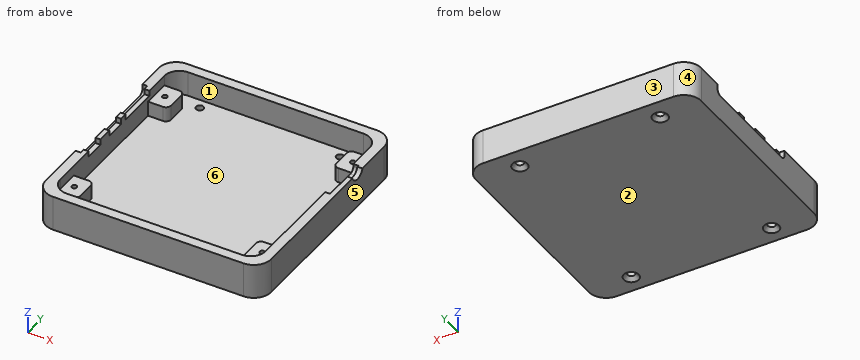
from build123d import *

# Parameters (mm, degrees)
CYLINDER005_R     = 1
CYLINDER005_DEPTH = 8
BOX014_W          = 8
BOX014_H          = 11
BOX014_DEPTH      = 6
FILLET006_R       = 2
CYLINDER006_R     = 1
CYLINDER006_DEPTH = 9
BOX013_W          = 8
BOX013_H          = 11
BOX013_DEPTH      = 6
FILLET005_R       = 2
CYLINDER004_R     = 1
CYLINDER004_DEPTH = 8
BOX011_W          = 8
BOX011_H          = 11
BOX011_DEPTH      = 6
FILLET004_R       = 2
CYLINDER003_R     = 1
CYLINDER003_DEPTH = 8
BOX009_W          = 8
BOX009_H          = 11
BOX009_DEPTH      = 6
FILLET003_R       = 2
BOX024_W          = 2
BOX024_H          = 45
BOX024_DEPTH      = 8
FILLET007_R       = 2
BOX023_W          = 6
BOX023_H          = 8
BOX023_DEPTH      = 3
CYLINDER008_R     = 1.5
CYLINDER008_DEPTH = 10
CYLINDER009_R     = 1.5
CYLINDER009_DEPTH = 10
CYLINDER010_R     = 1.5
CYLINDER010_DEPTH = 10
CYLINDER007_R     = 1.5
CYLINDER007_DEPTH = 10
BOX018_W          = 6
BOX018_H          = 8
BOX018_DEPTH      = 3
BOX015_W          = 16
BOX015_H          = 16
BOX015_DEPTH      = 2.25
CYLINDER002_R     = 3.5
CYLINDER002_DEPTH = 10.5
BOX010_W          = 2
BOX010_H          = 19
BOX010_DEPTH      = 8
FILLET002_R       = 2
BOX008_W          = 90
BOX008_H          = 90
BOX008_DEPTH      = 14
BOX006_W          = 82
BOX006_H          = 82
BOX006_DEPTH      = 82
FILLET001_R       = 6
BOX005_W          = 90
BOX005_H          = 90
BOX005_DEPTH      = 90
FILLET_R          = 7
CHAMFER_SIZE      = 1.5


with BuildPart() as cylinder002:
    # Cylinder005 → Cylinder005 (new body)
    with BuildSketch(Plane(origin=(82.5, 74.5, 4), x_dir=(1, 0, 0), z_dir=(0, 0, 1))):
        Circle(CYLINDER005_R)
    extrude(amount=CYLINDER005_DEPTH)


with BuildPart() as cut003:
    # Box014 → Box014 (new body)
    with BuildSketch(Plane(origin=(78, 8, 4), x_dir=(1, 0, 0), z_dir=(0, 0, 1))):
        with Locations((4, 5.5)):
            Rectangle(BOX014_W, BOX014_H)
    extrude(amount=BOX014_DEPTH)

    # Fillet006
    fillet006_edges = [cut003.edges().sort_by_distance(p)[0] for p in [
        (78, 8, 7),
        (78, 19, 7),
    ]]
    fillet(fillet006_edges, radius=FILLET006_R)


with BuildPart() as cut003_1:
    # Fillet006 placement: moved
    add(cut003.part.moved(Location((0, 61, 0))))

    # Cut003: cut Cylinder002
    add(cylinder002.part, mode=Mode.SUBTRACT)


with BuildPart() as cylinder003:
    # Cylinder006 → Cylinder006 (new body)
    with BuildSketch(Plane(origin=(82.5, 13.5, 4), x_dir=(1, 0, 0), z_dir=(0, 0, 1))):
        Circle(CYLINDER006_R)
    extrude(amount=CYLINDER006_DEPTH)


with BuildPart() as cut004:
    # Box013 → Box013 (new body)
    with BuildSketch(Plane(origin=(78, 8, 4), x_dir=(1, 0, 0), z_dir=(0, 0, 1))):
        with Locations((4, 5.5)):
            Rectangle(BOX013_W, BOX013_H)
    extrude(amount=BOX013_DEPTH)

    # Fillet005
    fillet005_edges = [cut004.edges().sort_by_distance(p)[0] for p in [
        (78, 8, 7),
        (78, 19, 7),
    ]]
    fillet(fillet005_edges, radius=FILLET005_R)

    # Cut004: cut Cylinder003
    add(cylinder003.part, mode=Mode.SUBTRACT)


with BuildPart() as cylinder001:
    # Cylinder004 → Cylinder004 (new body)
    with BuildSketch(Plane(origin=(7.5, 74.5, 4), x_dir=(1, 0, 0), z_dir=(0, 0, 1))):
        Circle(CYLINDER004_R)
    extrude(amount=CYLINDER004_DEPTH)


with BuildPart() as cut005:
    # Box011 → Box011 (new body)
    with BuildSketch(Plane(origin=(4, 8, 3), x_dir=(1, 0, 0), z_dir=(0, 0, 1))):
        with Locations((4, 5.5)):
            Rectangle(BOX011_W, BOX011_H)
    extrude(amount=BOX011_DEPTH)

    # Fillet004
    fillet004_edges = [cut005.edges().sort_by_distance(p)[0] for p in [
        (12, 8, 6),
        (12, 19, 6),
    ]]
    fillet(fillet004_edges, radius=FILLET004_R)


with BuildPart() as cut005_1:
    # Fillet004 placement: moved
    add(cut005.part.moved(Location((0, 61, 1))))

    # Cut005: cut Cylinder001
    add(cylinder001.part, mode=Mode.SUBTRACT)


with BuildPart() as cylinder:
    # Cylinder003 → Cylinder003 (new body)
    with BuildSketch(Plane(origin=(7.5, 13.5, 4), x_dir=(1, 0, 0), z_dir=(0, 0, 1))):
        Circle(CYLINDER003_R)
    extrude(amount=CYLINDER003_DEPTH)


with BuildPart() as cut006:
    # Box009 → Box009 (new body)
    with BuildSketch(Plane(origin=(4, 8, 3), x_dir=(1, 0, 0), z_dir=(0, 0, 1))):
        with Locations((4, 5.5)):
            Rectangle(BOX009_W, BOX009_H)
    extrude(amount=BOX009_DEPTH)

    # Fillet003
    fillet003_edges = [cut006.edges().sort_by_distance(p)[0] for p in [
        (12, 8, 6),
        (12, 19, 6),
    ]]
    fillet(fillet003_edges, radius=FILLET003_R)


with BuildPart() as cut006_1:
    # Fillet003 placement: moved
    add(cut006.part.moved(Location((0, 0, 1))))

    # Cut006: cut Cylinder
    add(cylinder.part, mode=Mode.SUBTRACT)


with BuildPart() as fillet007:
    # Box024 → Box024 (new body)
    with BuildSketch(Plane(origin=(0, 27, 10), x_dir=(1, 0, 0), z_dir=(0, 0, 1))):
        with Locations((1, 22.5)):
            Rectangle(BOX024_W, BOX024_H)
    extrude(amount=BOX024_DEPTH)

    # Fillet007
    fillet007_edges = [fillet007.edges().sort_by_distance(p)[0] for p in [
        (1, 27, 10),
        (1, 27, 18),
        (1, 72, 10),
        (1, 72, 18),
    ]]
    fillet(fillet007_edges, radius=FILLET007_R)


with BuildPart() as uart001:
    # Box023 → Box023 (new body)
    with BuildSketch(Plane(origin=(0, 43, 11.75), x_dir=(1, 0, 0), z_dir=(0, 0, 1))):
        with Locations((3, 4)):
            Rectangle(BOX023_W, BOX023_H)
    extrude(amount=BOX023_DEPTH)


with BuildPart() as cylinder005:
    # Cylinder008 → Cylinder008 (new body)
    with BuildSketch(Plane(origin=(17, 7, 0), x_dir=(1, 0, 0), z_dir=(0, 0, 1))):
        Circle(CYLINDER008_R)
    extrude(amount=CYLINDER008_DEPTH)


with BuildPart() as cylinder006:
    # Cylinder009 → Cylinder009 (new body)
    with BuildSketch(Plane(origin=(17, 82, 0), x_dir=(1, 0, 0), z_dir=(0, 0, 1))):
        Circle(CYLINDER009_R)
    extrude(amount=CYLINDER009_DEPTH)


with BuildPart() as cylinder007:
    # Cylinder010 → Cylinder010 (new body)
    with BuildSketch(Plane(origin=(73, 82, 0), x_dir=(1, 0, 0), z_dir=(0, 0, 1))):
        Circle(CYLINDER010_R)
    extrude(amount=CYLINDER010_DEPTH)


with BuildPart() as cylinder004:
    # Cylinder007 → Cylinder007 (new body)
    with BuildSketch(Plane(origin=(73, 7, 0), x_dir=(1, 0, 0), z_dir=(0, 0, 1))):
        Circle(CYLINDER007_R)
    extrude(amount=CYLINDER007_DEPTH)


with BuildPart() as power001:
    # Box018 → Box018 (new body)
    with BuildSketch(Plane(origin=(0, 29, 11.75), x_dir=(1, 0, 0), z_dir=(0, 0, 1))):
        with Locations((3, 4)):
            Rectangle(BOX018_W, BOX018_H)
    extrude(amount=BOX018_DEPTH)


with BuildPart() as sd001:
    # Box015 → Box015 (new body)
    with BuildSketch(Plane(origin=(0, 54, 11.75), x_dir=(1, 0, 0), z_dir=(0, 0, 1))):
        with Locations((8, 8)):
            Rectangle(BOX015_W, BOX015_H)
    extrude(amount=BOX015_DEPTH)


with BuildPart() as headphone001:
    # Cylinder002 → Cylinder002 (new body)
    with BuildSketch(Plane(origin=(80, 65, 15), x_dir=(0, 0, -1), z_dir=(1, 0, 0))):
        Circle(CYLINDER002_R)
    extrude(amount=CYLINDER002_DEPTH)


with BuildPart() as fillet002:
    # Box010 → Box010 (new body)
    with BuildSketch(Plane(origin=(86, 50, 11), x_dir=(1, 0, 0), z_dir=(0, 0, 1))):
        with Locations((1, 9.5)):
            Rectangle(BOX010_W, BOX010_H)
    extrude(amount=BOX010_DEPTH)

    # Fillet002
    fillet002_edges = [fillet002.edges().sort_by_distance(p)[0] for p in [
        (87, 50, 11),
        (87, 50, 19),
        (87, 69, 11),
        (87, 69, 19),
    ]]
    fillet(fillet002_edges, radius=FILLET002_R)


with BuildPart() as cube003:
    # Box008 → Box008 (new body)
    with BuildSketch(Plane.XY):
        with Locations((45, 45)):
            Rectangle(BOX008_W, BOX008_H)
    extrude(amount=BOX008_DEPTH)


with BuildPart() as fillet001:
    # Box006 → Box006 (new body)
    with BuildSketch(Plane.XY):
        with Locations((41, 41)):
            Rectangle(BOX006_W, BOX006_H)
    extrude(amount=BOX006_DEPTH)

    # Fillet001
    fillet001_edges = [fillet001.edges().sort_by_distance(p)[0] for p in [
        (0, 0, 41),
        (0, 41, 82),
        (0, 82, 41),
        (82, 0, 41),
        (82, 41, 82),
        (82, 82, 41),
        (41, 0, 82),
        (41, 82, 82),
    ]]
    fillet(fillet001_edges, radius=FILLET001_R)


with BuildPart() as fillet001_1:
    # Fillet001 placement: moved
    add(fillet001.part.moved(Location((4, 4, 4))))


with BuildPart() as bottom001:
    # Box005 → Box005 (new body)
    with BuildSketch(Plane.XY):
        with Locations((45, 45)):
            Rectangle(BOX005_W, BOX005_H)
    extrude(amount=BOX005_DEPTH)

    # Fillet
    fillet_edges = [bottom001.edges().sort_by_distance(p)[0] for p in [
        (0, 0, 45),
        (0, 45, 90),
        (0, 90, 45),
        (90, 0, 45),
        (90, 45, 90),
        (90, 90, 45),
        (45, 0, 90),
        (45, 90, 90),
    ]]
    fillet(fillet_edges, radius=FILLET_R)

    # Cut: cut Fillet001
    add(fillet001_1.part, mode=Mode.SUBTRACT)

    # Common: intersect Cube003
    add(cube003.part, mode=Mode.INTERSECT)

    # Cut001: cut Fillet002
    add(fillet002.part, mode=Mode.SUBTRACT)

    # Cut002: cut Headphone001
    add(headphone001.part, mode=Mode.SUBTRACT)

    # Cut007: cut sd001
    add(sd001.part, mode=Mode.SUBTRACT)

    # Cut008: cut power001
    add(power001.part, mode=Mode.SUBTRACT)

    # Cut009: cut Cylinder004
    add(cylinder004.part, mode=Mode.SUBTRACT)

    # Cut010: cut Cylinder007
    add(cylinder007.part, mode=Mode.SUBTRACT)

    # Cut011: cut Cylinder006
    add(cylinder006.part, mode=Mode.SUBTRACT)

    # Cut012: cut Cylinder005
    add(cylinder005.part, mode=Mode.SUBTRACT)

    # Cut013: cut uart001
    add(uart001.part, mode=Mode.SUBTRACT)

    # Cut014: cut Fillet007
    add(fillet007.part, mode=Mode.SUBTRACT)

    # Chamfer
    chamfer_edges = [bottom001.edges().sort_by_distance(p)[0] for p in [
        (15.5, 82, 0),
        (15.5, 7, 0),
        (71.5, 7, 0),
        (71.5, 82, 0),
    ]]
    chamfer(chamfer_edges, length=CHAMFER_SIZE)

    # Fusion: union Cut003, Cut004, Cut005, Cut006
    add(cut003_1.part)
    add(cut004.part)
    add(cut005_1.part)
    add(cut006_1.part)


with BuildPart() as bottom001_1:
    # Fusion placement: moved
    add(bottom001.part.moved(Location((0, 0, -20))))


solid = bottom001_1.part
Design review of the part built by this model. Coordinates are the model's own, in mm. Face numbers are marked on the shaded views. A direction names the side the tool comes from. Coordinates: 2 decimals unless noted, no trailing zeros. Loops run counter-clockwise (first coordinate to the right, second up) from the corner with the lowest first, then second, coordinate; pieces in that order, holes last. Notation, with made-up numbers: (62, 60.5) -> (101, 60.5) arc R20 cw to (101, 71.5) -> close; hole circle Ø2 at (-20, 21.5). An arc over 180 degrees is marked (long way). Use a Markdown table: item, result. Add a question column.
Item 1: We need section C-C, the plane x = 68. Write out the cut boundary in (y, z), and give its area (3 significant figures).
Item 2: Clearance check with flat-ended pins moving along their axes: P1, Ø1, axis at x = 2.5, z = -7, coming from the +Y side; P2, Ø4, axis at x = 6.5, y = 74, coming from the +Z side; P3, Ø1.6, axis at x = 3, z = -7.5, coming from the -Y side. State where each tip first meets the part, or that it passes through.
Item 3: Machinability: for the marked faces 1 and 2, which of the approach directions +Z, -Z, +X, -X, +Y, -Y give a long, thin tool a straight path to every point of the face, cutting with its end or side? Answer none if there is none.
Item 4: Wall thickness on L1, parallel to Y at x = 73, z = -16.5; L2, parallel to X at y = 82, z = -16.85; L3, parallel to X at y = 74.5, z = -12.05: over which ranges is each line inside the solid? List them lowest first. Write a range as from..to.
Item 5: We need section B-B, the plane y = 39.5. Write out the cut boundary in (x, z), and give its area (3 significant figures).
Item 6: The part is to be moulded in two halves that separate along X. For the marked faces 3, 4, 5 and 6, say which applies: +X half, -X half, draft (parallel to the pull), parting line (faces both ways), or undercut.
Item 7: We need section A-A, the plane x = 17. Write out the cut boundary in (y, z).
Numbers:
| question | item | result |
|---|---|---|
| 1 | outline | (0, -20) -> (90, -20) -> (90, -6) -> (86, -6) -> (86, -16) -> (4, -16) -> (4, -6) -> (0, -6) -> close |
| 1 | area | 440 mm^2 |
| 2 | P1 | stops at y = 88.74 |
| 2 | P2 | stops at z = -10 |
| 2 | P3 | stops at y = 0.77 |
| 3 | face 1 | +Z |
| 3 | face 2 | -Z, +X, -X, +Y, -Y |
| 4 | L1 | y = 0..5.5, 8.5..80.5, 83.5..90 |
| 4 | L2 | x = 0..15.5, 18.5..71.5, 74.5..90 |
| 4 | L3 | x = 0..6.5, 8.5..12, 78..81.5, 83.5..90 |
| 5 | outline | (0, -20) -> (90, -20) -> (90, -6) -> (86, -6) -> (86, -16) -> (4, -16) -> (4, -6) -> (2, -6) -> (2, -10) -> (0, -10) -> close |
| 5 | area | 432 mm^2 |
| 6 | face 3 | draft |
| 6 | face 4 | -X half |
| 6 | face 5 | +X half |
| 6 | face 6 | undercut |
| 7 | outline | (0, -20) -> (4, -20) -> (5.5, -18.5) -> (5.5, -16) -> (4, -16) -> (4, -6) -> (0, -6) -> close; (8.5, -18.5) -> (10, -20) -> (79, -20) -> (80.5, -18.5) -> (80.5, -16) -> (8.5, -16) -> close; (83.5, -18.5) -> (85, -20) -> (90, -20) -> (90, -6) -> (86, -6) -> (86, -16) -> (83.5, -16) -> close |
